Can you work these out from the model? Positions are in its coordinate system, mm. Coordinates: 2 decimals unless noted, no trailing zeros. Loops run counter-clockwise (first coordinate to the right, second up) from the corner with the lowest first, then second, coordinate; pieces in that order, holes last. Notation, with made-up numbers: (32.25, 78.25) -> (55.25, 78.25) arc R17 ccw to (55.25, 92.25) -> close; hole circle Ø11 at (62, -28). An arc over 180 degrees is marked (long way). Put each result on its own line as item: value. Start each with the question number.
Item 1: If we section it at D-D on x = -15: Please give me the cut outline in (y, z).
Item 2: We'd pull the mould along X, two halves only. Please class faces 1 (the flat face through (-22.15, 0.02, 53.38)), 2 (the flat face through (0, 1.588, 8)), 3 (the cylindrical face through (-3.84, -0.02, 58.31)): pulls with the +X half, pulls with the -X half, needs draft (parallel to the pull), parting line crosses it, or undercut.
Item 3: If we section it at C-C on y = 0.1: State how many separate pieces and enclosed holes the cut face has, plus the area to 3 significant figures.
Item 4: Please list where these lines run through material, in increasing order: L1, parallel to X at y = -0.55, z = 30; L2, parallel to X at y = 1.2, z = 31.5; L3, parallel to Z at x = -27.5, y = 0.95. Write a range as from..to.
Item 5: If we section it at B-B on z = -20: Please give me the cut outline in (x, y).
Item 6: If we section it at A-A on x = -4: Please give me the cut outline in (y, z).
```python
from build123d import *

# Parameters (mm, degrees)
SKETCH1_W            = 65
SKETCH1_H            = 90
SKETCH1_W_2          = 23
SKETCH1_H_2          = 17
BOSS_EXTRUDE1_DEPTH  = 1.5875
M2_CLEARANCE_HOLE1_D = 2.4
M4_CLEARANCE_HOLE1_D = 4.5
M4_CLEARANCE_HOLE2_D = 4.5
M4_CLEARANCE_HOLE3_D = 4.5


with BuildPart() as part:
    # Sketch1 → Boss-Extrude1 (new body, symmetric)
    with BuildSketch(Plane(origin=(0, 0, 0), x_dir=(1, 0, 0), z_dir=(0, 1, 0))):
        Polygon((-32.5, -45), (-11.5, -62), (-11.5, -45), align=None)
        Polygon((11.5, -45), (11.5, -62), (32.5, -45), align=None)
        Rectangle(SKETCH1_W, SKETCH1_H)
        with Locations((0, -53.5)):
            Rectangle(SKETCH1_W_2, SKETCH1_H_2)
    extrude(amount=BOSS_EXTRUDE1_DEPTH, both=True)

    # M2 Clearance Hole1 (through all)
    with Locations(Plane(origin=(0, 1.5875, 0), x_dir=(1, 0, 0), z_dir=(0, 1, 0))):
        with Locations((-4, -59.5), (4, -59.5), (4, -47.5), (-4, -47.5)):
            Hole(M2_CLEARANCE_HOLE1_D / 2)

    # M4 Clearance Hole1 (through all)
    with Locations(Plane(origin=(0, 1.5875, 0), x_dir=(1, 0, 0), z_dir=(0, 1, 0))):
        with Locations((-27.5, 20), (27.5, 20), (27.5, -30), (-27.5, -30)):
            Hole(M4_CLEARANCE_HOLE1_D / 2)

    # M4 Clearance Hole2 (through all)
    with Locations(Plane(origin=(0, 1.5875, 0), x_dir=(1, 0, 0), z_dir=(0, 1, 0))):
        with Locations((-19.5, -11.575), (-19.5, 3.425), (5.5, 3.425), (5.5, -11.575)):
            Hole(M4_CLEARANCE_HOLE2_D / 2)

    # M4 Clearance Hole3 (through all)
    with Locations(Plane(origin=(0, -1.5875, 0), x_dir=(-1, 0, 0), z_dir=(0, -1, 0))):
        with Locations((-15, 37.6), (15, 37.6)):
            Hole(M4_CLEARANCE_HOLE3_D / 2)


solid = part.part
```
Solutions:
1. outline: (-1.59, -45) -> (1.59, -45) -> (1.59, -39.85) -> (-1.59, -39.85) -> close; (-1.59, -35.35) -> (1.59, -35.35) -> (1.59, 59.17) -> (-1.59, 59.17) -> close
2. face 1: pulls with the -X half
2. face 2: needs draft
2. face 3: undercut
3. separate pieces: 1
3. enclosed holes: 14
3. area: 6,420 mm^2
4. L1: -32.5..-29.75, -25.25..25.25, 29.75..32.5
4. L2: -32.5..-29.18, -25.82..25.82, 29.18..32.5
4. L3: -45..-22.25, -17.75..27.75, 32.25..49.05
5. outline: (-32.5, -1.59) -> (-29.75, -1.59) -> (-29.75, 1.59) -> (-32.5, 1.59) -> close; (-25.25, -1.59) -> (25.25, -1.59) -> (25.25, 1.59) -> (-25.25, 1.59) -> close; (29.75, -1.59) -> (32.5, -1.59) -> (32.5, 1.59) -> (29.75, 1.59) -> close
6. outline: (-1.59, -45) -> (1.59, -45) -> (1.59, 46.3) -> (-1.59, 46.3) -> close; (-1.59, 48.7) -> (1.59, 48.7) -> (1.59, 58.3) -> (-1.59, 58.3) -> close; (-1.59, 60.7) -> (1.59, 60.7) -> (1.59, 62) -> (-1.59, 62) -> close
